Autodesk Inventor part; units mm, degrees
ref_plane "YZ Plane" through (0, 0, 0) normal (1, 0, 0) x (0, 1, 0)
ref_plane "XZ Plane" through (0, 0, 0) normal (0, 1, 0) x (-1, 0, 0)
ref_plane "XY Plane" through (0, 0, 0) normal (0, 0, 1) x (1, 0, 0)
sketch "Sketch1" plane through (0, 0, 0) normal (0, 1, 0) x (-1, 0, 0)
  line L0 (-25.4, 76.2) -> (25.4, 76.2)
  line L1 (-50.8, 50.8) -> (-50.8, -50.8)
  line L2 (50.8, 76.2) -> (-50.8, 76.2)
  line L3 (-25.4, -76.2) -> (25.4, -76.2)
  line L4 (50.8, -50.8) -> (50.8, 50.8)
  arc A0 (50.8, 50.8) -> (25.4, 76.2) centre (25.4, 50.8) ccw
  arc A1 (25.4, -76.2) -> (50.8, -50.8) centre (25.4, -50.8) ccw
  arc A2 (-50.8, -50.8) -> (-25.4, -76.2) centre (-25.4, -50.8) ccw
  arc A3 (-25.4, 76.2) -> (-50.8, 50.8) centre (-25.4, 50.8) ccw
  circle A4 centre (-25.4, 50.8) radius 25.4
  circle A5 centre (-25.4, -50.8) radius 25.4
  circle A6 centre (-50.8, 0) radius 31.3961
  circle A7 centre (-82.1961, 0) radius 50.8
  point P0 (-36.7592, 28.0815)
  point P1 (-36.7592, -28.0815)
  point P2 (-50.8, 31.3961)
  point P3 (-50.8, -31.3961)
  point P4 (-44.332, 33.8667)
  point P5 (-44.332, -33.8667)
  dimension "d6" = 101.6
  dimension "d21" = 25.4
extrude "Extrusion5" add sketch "Sketch1" along normal blind 3 contours A4 A3 | L0 A0 L4 A1 L3 A5 A6 A4 | A4 A6 A7 | A6 A7 | A5 A2 | A7 A6 A5
sketch "Sketch3" plane through (0, 3, 0) normal (0, 1, 0) x (1, 0, 0)
  arc A0 (-50.8, -50.8) -> (-25.4, -76.2) centre (-25.4, -50.8) ccw
  arc A1 (-50.8, -50.8) -> (-25.4, -76.2) centre (-25.4, -50.8) ccw
  arc A2 (-25.4, 76.2) -> (-50.8, 50.8) centre (-25.4, 50.8) ccw
  line L0 (-50.8, 50.8) -> (-50.8, -50.8)
  arc A3 (-25.4, 76.2) -> (-50.8, 50.8) centre (-25.4, 50.8) ccw
  arc A4 (25.4, -76.2) -> (44.332, -33.8667) centre (25.4, -50.8) ccw
  arc A5 (25.4, -76.2) -> (44.332, -33.8667) centre (25.4, -50.8) ccw
  arc A6 (44.332, 33.8667) -> (44.332, -33.8667) centre (82.1961, 0) ccw
  arc A7 (44.332, 33.8667) -> (44.332, -33.8667) centre (82.1961, 0) ccw
  arc A8 (44.332, 33.8667) -> (25.4, 76.2) centre (25.4, 50.8) ccw
  arc A9 (44.332, 33.8667) -> (25.4, 76.2) centre (25.4, 50.8) ccw
  line L1 (-50.8, -50.8) -> (-50.8, 50.8)
  line L2 (-25.4, -76.2) -> (25.4, -76.2)
  line L3 (-25.4, -76.2) -> (25.4, -76.2)
  line L4 (-25.4, 76.2) -> (25.4, 76.2)
  line L5 (-25.4, 76.2) -> (25.4, 76.2)
  line L6 (25.4, 76.2) -> (-25.4, 76.2)
  line L7 (25.4, 76.2) -> (-25.4, 76.2)
  line L8 (25.4, 76.2) -> (-25.4, 76.2)
  arc A10 (-48.8, -50.8) -> (-25.4, -74.2) centre (-25.4, -50.8) ccw
  line L9 (-25.4, -74.2) -> (25.4, -74.2)
  arc A11 (25.4, -74.2) -> (42.8413, -35.2) centre (25.4, -50.8) ccw
  arc A12 (42.8413, 35.2) -> (42.8413, -35.2) centre (82.1961, 0) ccw
  arc A13 (42.8413, 35.2) -> (25.4, 74.2) centre (25.4, 50.8) ccw
  line L10 (25.4, 74.2) -> (-25.4, 74.2)
  arc A14 (-25.4, 74.2) -> (-48.8, 50.8) centre (-25.4, 50.8) ccw
  line L11 (-48.8, 50.8) -> (-48.8, -50.8)
  point P0 (0, 0)
  dimension "d28" = 2
extrude "Extrusion6" add sketch "Sketch3" along normal blind 2
hole "Hole2" at (-25.4, 0, 50.8) at (25.4, 0, 50.8) at (25.4, 0, -50.8) at (-25.4, 0, -50.8) direction (0, 1, 0) diameter 3 depth 25.4 tip angle 118
properties part number "ControllerBottom"
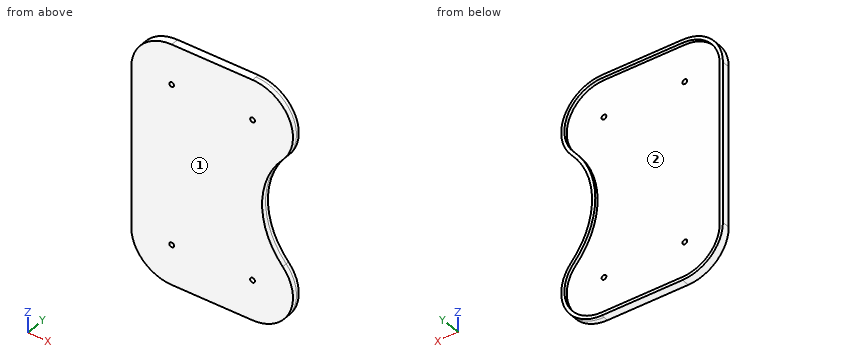
CAD build for the part. Positions are in the model's coordinates, mm. Face numbers are marked on the shaded views. Coordinates: 2 decimals unless noted, no trailing zeros. Write each loop counter-clockwise with the first axis right and the second up, starting at its lowest first coordinate (ties: lowest second). Pieces come first, ordered by that corner, then holes. Notation, with made-up numbers: (64.25, 9) - (81.25, 9) arc R25 cw to (81.25, 21) - close; hole circle Ø9 at (-37.75, 64). An arc over 180 degrees is marked (long way). Use a Markdown table: item, result. Add a question column.
Item 1: Drill centre lines: L1, parallel to X at y = 2.45, z = 50.8; L2, parallel to Z at x = 25.4, y = 1.65; L3, parallel to Z at x = -3, y = 3.1. Where is each one in solid material? Low to high. Write a range as from..to.
Item 2: Band-saw the part on A-A, the plane y = 2.25. Give the cut face in (x, z).
Item 3: Band-saw the part on C-C, the plane z = -39.5. Give the cut face in (x, y).
Item 4: Flat gauge pins, fed straight in: pin 1 (1.5 mm diameter, centred on x = -23, z = 28, fed in from +Y); pin 2 (2 mm diameter, centred on y = 3.5, z = -61, fed in from +X); pin 3 (1 mm diameter, centred on y = 4, z = -4, fed in from +X). Where does each tip first touch, or does it go through?
Item 5: Mould opens along X. For the marked faces 1 and 2 say: pulls with the +X half, pulls with the -X half, needs draft (parallel to the pull), parting line crosses it, or undercut.
Item 6: Band-saw the part on B-B, the plane x = -10.5. Give the cut face in (y, z), and give its area (3 significant figures).
Numbers:
| question | item | result |
|---|---|---|
| 1 | L1 | -50.8..-26.9, -23.9..23.9, 26.9..50.8 |
| 1 | L2 | -76.2..-52.3, -49.3..49.3, 52.3..76.2 |
| 1 | L3 | -76.2..-74.2, 74.2..76.2 |
| 2 | outline | (-50.8, -50.8) arc R25.4 ccw to (-25.4, -76.2) - (25.4, -76.2) arc R25.4 ccw to (44.33, -33.87) arc R50.8 cw to (44.33, 33.87) arc R25.4 ccw to (25.4, 76.2) - (-25.4, 76.2) arc R25.4 ccw to (-50.8, 50.8) - close; hole circle Ø3 at (-25.4, -50.8); hole circle Ø3 at (-25.4, 50.8); hole circle Ø3 at (25.4, -50.8); hole circle Ø3 at (25.4, 50.8) |
| 3 | outline | (-50.8, 0) - (48.15, 0) - (48.15, 5) - (45.89, 5) - (45.89, 3) - (-48.8, 3) - (-48.8, 5) - (-50.8, 5) - close |
| 4 | pin 1 | y = 3 |
| 4 | pin 2 | x = 49.08 |
| 4 | pin 3 | x = 31.6 |
| 5 | face 1 | needs draft |
| 5 | face 2 | undercut |
| 6 | outline | (0, -76.2) - (5, -76.2) - (5, -74.2) - (3, -74.2) - (3, 74.2) - (5, 74.2) - (5, 76.2) - (0, 76.2) - close |
| 6 | area | 465 mm2 |
